```python
from build123d import *

# Parameters (mm, degrees)
STOCK_MASTER_SKETCH_002_1_START     = 413
STOCK_MASTER_SKETCH_002_1_OUTLINE_W = 75
STOCK_MASTER_SKETCH_002_1_OUTLINE_H = 75
STOCK_MASTER_SKETCH_002_1_OUTLINE_R = 2.5
STOCK_MASTER_SKETCH_002_1_DEPTH     = 5
FILLET1_R                           = 3


# Read off the part's stored shape, not the designer's step: Stock-master_sketch_002-1
with BuildPart() as part:
    # Stock-master_sketch_002-1 outline → Stock-master_sketch_002-1 (new body)
    with BuildSketch(Plane.YZ.offset(STOCK_MASTER_SKETCH_002_1_START)):
        with Locations((0, 1880)):
            Rectangle(STOCK_MASTER_SKETCH_002_1_OUTLINE_W, STOCK_MASTER_SKETCH_002_1_OUTLINE_H)
        with Locations((-21.25, 1860)):
            Circle(STOCK_MASTER_SKETCH_002_1_OUTLINE_R, mode=Mode.SUBTRACT)
        with Locations((21.25, 1860)):
            Circle(STOCK_MASTER_SKETCH_002_1_OUTLINE_R, mode=Mode.SUBTRACT)
        with Locations((-21.25, 1880)):
            Circle(STOCK_MASTER_SKETCH_002_1_OUTLINE_R, mode=Mode.SUBTRACT)
        with Locations((-21.25, 1900)):
            Circle(STOCK_MASTER_SKETCH_002_1_OUTLINE_R, mode=Mode.SUBTRACT)
        with Locations((21.25, 1880)):
            Circle(STOCK_MASTER_SKETCH_002_1_OUTLINE_R, mode=Mode.SUBTRACT)
        with Locations((21.25, 1900)):
            Circle(STOCK_MASTER_SKETCH_002_1_OUTLINE_R, mode=Mode.SUBTRACT)
    extrude(amount=STOCK_MASTER_SKETCH_002_1_DEPTH)

    # Fillet1
    fillet1_edges = [part.edges().sort_by_distance(p)[0] for p in [
        (415.5, 37.5, 1917.5),
        (415.5, 37.5, 1842.5),
        (415.5, -37.5, 1842.5),
        (415.5, -37.5, 1917.5),
    ]]
    fillet(fillet1_edges, radius=FILLET1_R)


solid = part.part
```
CAD build for the part. Positions are in the model's coordinates, mm. Coordinates: 2 decimals unless noted, no trailing zeros. Order: outer loops, then holes, each group sorted by start corner. A loop starts at its lowest first (then second) coordinate and runs counter-clockwise, first axis right, second up. Notation, with made-up numbers: M 1,-23.5 L 18,-23.5 A31 cw 18,10.5 Z; hole C 51.5,59.5 d1. An arc over 180 degrees is marked long. Answer as CSV lines item,"result".
1) Cut at B-B (x = 414.5). List the corners of the cut face in (y, z).
Verdict:
outline,"M -37.5,1845.5 A3 ccw -34.5,1842.5 L 34.5,1842.5 A3 ccw 37.5,1845.5 L 37.5,1914.5 A3 ccw 34.5,1917.5 L -34.5,1917.5 A3 ccw -37.5,1914.5 Z; hole C -21.25,1860 d5; hole C -21.25,1880 d5; hole C -21.25,1900 d5; hole C 21.25,1860 d5; hole C 21.25,1880 d5; hole C 21.25,1900 d5"
2) Cut at A-A (y = -21.25). List the corners of the cut face in (x, z).
Verdict:
outline,"M 413,1842.5 L 418,1842.5 L 418,1857.5 L 413,1857.5 Z; M 413,1862.5 L 418,1862.5 L 418,1877.5 L 413,1877.5 Z; M 413,1882.5 L 418,1882.5 L 418,1897.5 L 413,1897.5 Z; M 413,1902.5 L 418,1902.5 L 418,1917.5 L 413,1917.5 Z"
3) Cut at C-C (z = 1900). List the corners of the cut face in (x, y).
Verdict:
outline,"M 413,-37.5 L 418,-37.5 L 418,-23.75 L 413,-23.75 Z; M 413,-18.75 L 418,-18.75 L 418,18.75 L 413,18.75 Z; M 413,23.75 L 418,23.75 L 418,37.5 L 413,37.5 Z"
4) Mould opens along Z. For faces 1 (the cylindrical face through (415.54, 36.6, 1843.36)), 2 (the flat face through (418, -1, 1881)), 3 (the cylindrical face through (415.46, 20.92, 1882.48)) say: released by +Z, released by -Z, zero draft, split by the parting line, or undercut.
Verdict:
face 1,"released by -Z"
face 2,"zero draft"
face 3,"undercut"
5) Flat gauge pin, fed straight in: P1, Ø4, axis at y = -21.25, z = 1860, coming from the -X side (3 decimals). Where does the tip first touch, or does it go through?
Verdict:
P1,"through"
6) Drill centre lines: L1, parallel to Z at x = 415.5, y = -21.25; L2, parallel to Y at x = 415.8, z = 1880; L3, parallel to Y at x = 414.45, z = 1861. Where is each one in solid material? Low to high. Write a range as from..to.
Verdict:
L1,"1842.5..1857.5, 1862.5..1877.5, 1882.5..1897.5, 1902.5..1917.5"
L2,"-37.5..-23.75, -18.75..18.75, 23.75..37.5"
L3,"-37.5..-23.54, -18.96..18.96, 23.54..37.5"
